Read the model definition and answer for the solid it produces. Units are mm, in the model's axes. Face numbers are marked on the shaded views. A direction names the side the tool comes from. Round coordinates to 2 decimals unless told otherwise and drop trailing zeros. Loops run counter-clockwise (first coordinate to the right, second up) from the corner with the lowest first, then second, coordinate; pieces in that order, holes last. Notation, with made-up numbers: M 84,14.25 L 138,14.25 A22 cw 138,31.25 Z; hole C 32,20 d2. An arc over 180 degrees is marked long. Write each question's results on one line, items separated by ' | '.
```python
from build123d import *

# Parameters (mm, degrees)
SKETCH_1_R          = 17.9
EXTRUDE_1_DEPTH     = 44
SKETCH_2_R          = 18.5
EXTRUDE_2_DEPTH     = 28
SKETCH_3_R          = 6
EXTRUDE_3_DEPTH     = 6
SKETCH_4_R          = 3
EXTRUDE_4_DEPTH     = 15
CUT_EXTRUDE_START   = -12
CUT_EXTRUDE_1_DEPTH = 12
M3X0_5_1_D          = 2.5
M3X0_5_1_DEPTH      = 8.5
M3X0_5_1_TIP        = 0.751075774
CHAMFER_1_SIZE      = 1
CHAMFER_2_SIZE      = 1
CHAMFER_3_SIZE      = 1


with BuildPart() as part:
    # ｽｹｯﾁ1 → ﾎﾞｽ - 押し出し1 (new body)
    with BuildSketch(Plane.XY):
        Circle(SKETCH_1_R)
    extrude(amount=EXTRUDE_1_DEPTH)

    # ｽｹｯﾁ2 → ﾎﾞｽ - 押し出し2 (add)
    with BuildSketch(Plane.XY.offset(44)):
        Circle(SKETCH_2_R)
    extrude(amount=EXTRUDE_2_DEPTH)

    # ｽｹｯﾁ3 → ﾎﾞｽ - 押し出し3 (add)
    with BuildSketch(Plane.XY.offset(72)):
        with Locations((0, 7)):
            Circle(SKETCH_3_R)
    extrude(amount=EXTRUDE_3_DEPTH)

    # ｽｹｯﾁ4 → ﾎﾞｽ - 押し出し4 (add)
    with BuildSketch(Plane.XY.offset(78)):
        with Locations((0, 7)):
            Circle(SKETCH_4_R)
    extrude(amount=EXTRUDE_4_DEPTH)

    # ｽｹｯﾁ5 → ｶｯﾄ - 押し出し1 (cut)
    with BuildSketch(Plane.XY.offset(93).offset(CUT_EXTRUDE_START)):
        with BuildLine():
            ThreePointArc((1.658312395, 9.5), (0, 10), (-1.658312395, 9.5))
            Line((-1.658312395, 9.5), (0, 9.5))
            Line((0, 9.5), (1.658312395, 9.5))
        make_face()
    extrude(amount=CUT_EXTRUDE_1_DEPTH, mode=Mode.SUBTRACT)

    # M3x0.5 ねじ穴1
    with Locations(Plane(origin=(-15.75, 0, 72), x_dir=(1, 0, 0), z_dir=(0, 0, 1))):
        with Locations((0, 0), (7.875, -13.63990011), (23.625, -13.63990011), (31.5, 0), (23.625, 13.63990011), (7.875, 13.63990011)):
            Hole(M3X0_5_1_D / 2, depth=M3X0_5_1_DEPTH)
            with Locations((0, 0, -(M3X0_5_1_DEPTH + M3X0_5_1_TIP / 2))):  # 118° drill point
                Cone(0, M3X0_5_1_D / 2, M3X0_5_1_TIP, mode=Mode.SUBTRACT)

    # 面取り1
    # the kernel refuses this chamfer: 1 mm, written as the material it takes off along each edge
    with BuildSketch(Plane(origin=(0, 7, 93), x_dir=(0.27051002147704706, 0.9627171590246472, 0), z_dir=(0.9627171590246472, -0.27051002147704706, 0))) as chamfer_1_piece_1:
        Polygon((3, -CHAMFER_1_SIZE), (3 - CHAMFER_1_SIZE, 0), (3, 0), align=None)
    revolve(axis=Axis((0, 7, 93), (0, 0, 1)), revolution_arc=285.694618346, mode=Mode.SUBTRACT)
    with BuildSketch(Plane(origin=(0, 7, 93), x_dir=(1, 0, 0), z_dir=(0, -1, 0))) as chamfer_1_piece_2:
        Polygon((3, -CHAMFER_1_SIZE), (3 - CHAMFER_1_SIZE, 0), (3, 0), align=None)
    revolve(axis=Axis((0, 7, 93), (0, 0, 1)), revolution_arc=105.565976033, mode=Mode.SUBTRACT)

    # 面取り2
    chamfer_2_edges = [part.edges().sort_by_distance(p)[0] for p in [
        (-6, 7, 78),
    ]]
    chamfer(chamfer_2_edges, length=CHAMFER_2_SIZE)

    # 面取り3
    chamfer_3_edges = [part.edges().sort_by_distance(p)[0] for p in [
        (-17.9, 0, 0),
    ]]
    chamfer(chamfer_3_edges, length=CHAMFER_3_SIZE)


solid = part.part
```
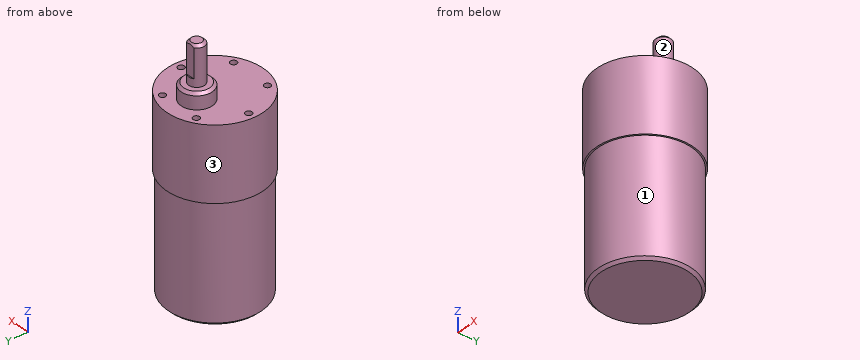
1. Find section B-B, the plane z = 10.5. Give the vertices of the cut face in (x, y), then the cut area to 3 significant figures.
Completed:
outline: C 0,0 d35.8 | area: 1,010 mm2
2. Find section A-A, the plane z = 67. Give the vertices of the cut face in (x, y) (3 decimals).
Completed:
outline: C 0,0 d37; hole C -15.75,0 d2.5; hole C -7.875,-13.64 d2.5; hole C -7.875,13.64 d2.5; hole C 7.875,-13.64 d2.5; hole C 7.875,13.64 d2.5; hole C 15.75,0 d2.5
3. Which of the six approach directions +Z, -Z, +X, -X, +Y, -Y give full straight-line access (tool end or side, diameter ignored) to the marked faces 1, 2 and 3?
Completed:
face 1: -Z | face 2: +Z | face 3: +Z, -Z
4. Find the intervals of material crossed by L1, parallel to Z at x = -11.5, y = -11; L2, parallel to Y at x = 15, z = 67; L3, parallel to Y at x = -0.5, z = 6.5, in increasing order.
Completed:
L1: z = 0 to 72 | L2: y = -10.83 to -1, 1 to 10.83 | L3: y = -17.89 to 17.89
5. Given P1, Ø4, axis at x = -5.5, z = 32, coming from the -Y side; P2, Ø18.5, axis at x = 7, y = -2.5, coming from the +Z side; P3, Ø2, axis at x = -9.5, y = 0, coming from the -Z side; P4, Ø4, axis at x = -14, z = 13.5, coming from the +Y side, each flat-ended and moving along its own axis, determine where each tip first touches the part or whether it passes through.
Completed:
P1: stops at y = -17.55 | P2: stops at z = 92.45 | P3: stops at z = 0 | P4: stops at y = 13.28
